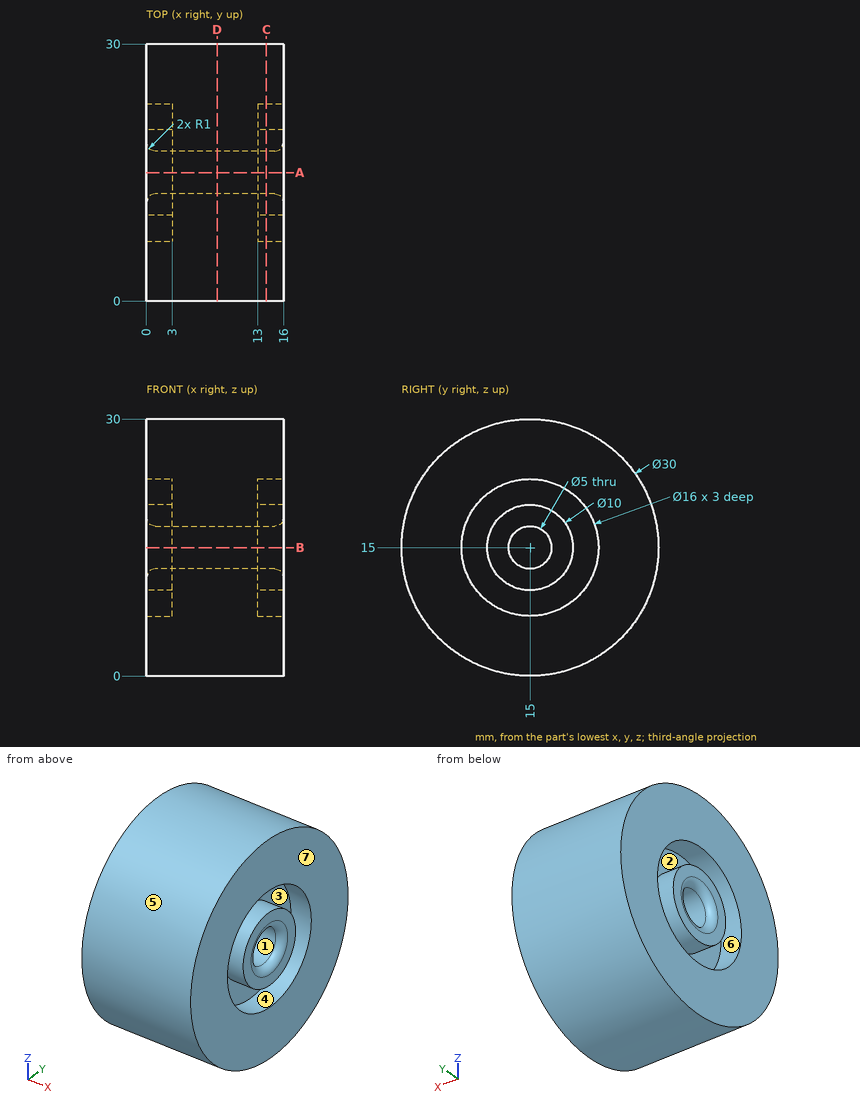
The drawing under review shows one solid part. Ordinate dimensions are in mm from its lowest x, y, z. A direction names the side the tool comes from. Round coordinates to 2 decimals unless told otherwise and drop trailing zeros. Write each loop counter-clockwise with the first axis right and the second up, starting at its lowest first coordinate (ties: lowest second). Pieces come first, ordered by that corner, then holes.
(1) Wall thickness on L1, parallel to Y at x = 1.9, z = 15; L2, parallel to Z at x = 15.1, y = 15; L3, parallel to Y at x = 9.25, z = 15: over which ranges is each line inside the solid? List them lowest first.
(2) Machinability: for the marked faces 1, 2 and 3, which of the approach directions +Z, -Z, +X, -X, +Y, -Y give a long, thin tool a straight path to every point of the face, cutting with its end or side? Answer none if there is none.
(3) We need section A-A on y = 15. Give the boundary of the cut face in (x, z), and give its area (3 significant figures).
(4) We need section D-D on x = 8.25. Give the boundary of the cut face in (y, z), and give its area (3 significant figures).
(5) We need section C-C on x = 14. Give the boundary of the cut face in (y, z), and give its area (3 significant figures).
(6) Insertion check: pin 1 (1 mm diameter, centred on x = 14, y = 4.5, fed in from -Z); pin 2 (6 mm diameter, centred on y = 15, z = 15, fed in from +X). Each pin has a flat end and moves straight along its axis. Give the tip position at first contact, or say it passes through.
(7) Mouldability with a two-part tool opening along Y and no side actions: class the marked faces 4, 5, 6 and 7 as +Y half, -Y half, draft (parallel to the pull), parting line (faces both ways), or undercut.
Findings below:
1. L1: y = 0 to 7, 10 to 12.5, 17.5 to 20, 23 to 30
1. L2: z = 0 to 7, 10 to 12.49, 17.51 to 20, 23 to 30
1. L3: y = 0 to 12.5, 17.5 to 30
2. face 1: +X, -X
2. face 2: -X
2. face 3: +X
3. outline: (0, 0) - (16, 0) - (16, 7) - (13, 7) - (13, 10) - (16, 10) - (16, 11.5) arc R1 ccw to (15, 12.5) - (1, 12.5) arc R1 ccw to (0, 11.5) - (0, 10) - (3, 10) - (3, 7) - (0, 7) - close; (0, 18.5) arc R1 ccw to (1, 17.5) - (15, 17.5) arc R1 ccw to (16, 18.5) - (16, 20) - (13, 20) - (13, 23) - (16, 23) - (16, 30) - (0, 30) - (0, 23) - (3, 23) - (3, 20) - (0, 20) - close
3. area: 363 mm2
4. outline: circle Ø30 at (15, 15); hole circle Ø5 at (15, 15)
4. area: 687 mm2
5. outline: circle Ø30 at (15, 15); circle Ø10 at (15, 15); hole circle Ø16 at (15, 15); hole circle Ø5 at (15, 15)
5. area: 565 mm2
6. pin 1: stops at z = 3.82
6. pin 2: stops at x = 15.87
7. face 4: undercut
7. face 5: parting line
7. face 6: undercut
7. face 7: draft
